Geometry: final body of the model. Coordinates: model frame, mm. Give positions to 0.01 mm unless a question says otherwise; leave off trailing zeros. Write each loop counter-clockwise with the first axis right and the second up, starting at its lowest first coordinate (ties: lowest second). Pieces come first, ordered by that corner, then holes. Notation, with made-up numbers: M 52,40.25 L 101,40.25 A10 cw 101,53.25 Z; hole C 8,73 d3. An arc over 180 degrees is marked long. Use one line per item in the form item = value. Start each with the question number.
Item 1: Section query B-B on x = -2.25. Return loops of the section in (y, z).
Item 2: Section query C-C on x = -3. Return loops of the section in (y, z).
Item 3: Contact query for a flat-ended pin moving along its axis: P1, Ø1, axis at x = -2, z = -3.5, coming from the -Y side. Output: stop coordinate, or through.
Item 4: Material intervals for line 1 along X through (y, z) = (9, 1.25); line 2 along Y through (x, z) = (-3, -4.5); line 3 along X through (y, z) = (8.75, -3.75), sorted ascending. Write a range as from..to.
Item 5: Section query A-A on z = -2.25. Return loops of the section in (x, y).
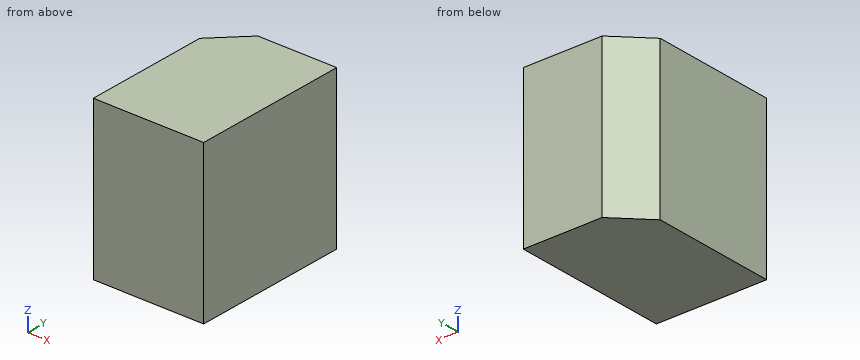
Autodesk Inventor part; units mm, degrees
ref_plane "YZ Plane" through (0, 0, 0) normal (1, 0, 0) x (0, 1, 0)
ref_plane "XZ Plane" through (0, 0, 0) normal (0, 1, 0) x (-1, 0, 0)
ref_plane "XY Plane" through (0, 0, 0) normal (0, 0, 1) x (1, 0, 0)
sketch "スケッチ1" plane through (0, 0, 0) normal (0, 1, 0) x (-1, 0, 0)
  line L0 (3.5, 5) -> (-3.5, 5)
  line L1 (-3.5, 5) -> (-3.5, -5)
  line L2 (-3.5, -5) -> (3.5, -5)
  line L3 (3.5, -5) -> (3.5, 5)
  line L4 (3.5, 5) -> (-3.5, -5) construction
  line L5 (-3.5, 5) -> (3.5, -5) construction
  point P0 (0, 0)
  dimension "d0" = 10
  dimension "d1" = 7
extrude "押し出し1" add sketch "スケッチ1" along normal blind 10
chamfer "面取り1" distance 2 angle 45 1 edges at (-3.5, 10, 0)
properties part number "terminalblock"
Answer sheet:
q1.outline = M 0,-5 L 9.25,-5 L 9.25,5 L 0,5 Z
q2.outline = M 0,-5 L 8.5,-5 L 8.5,5 L 0,5 Z
q3.P1 = 0
q4.line_1 = -2.5..3.5
q4.line_2 = 0..8.5
q4.line_3 = -2.75..3.5
q5.outline = M -3.5,0 L 3.5,0 L 3.5,10 L -1.5,10 L -3.5,8 Z
